Verification items for the finished model (mm, model axes). Face numbers are marked on the shaded views. Round coordinates to 2 decimals unless told otherwise and drop trailing zeros. Order: outer loops, then holes, each group sorted by start corner. A loop starts at its lowest first (then second) coordinate and runs counter-clockwise, first axis right, second up. Notation, with made-up numbers: (41, 74) -> (80, 74) arc R15 cw to (80, 86) -> close; hole circle Ø9 at (-11.75, 23). An arc over 180 degrees is marked (long way). Return JSON: item names as keys, results as strings. Group by question number.
Item 1: Sectioned sample at B-B on x = 32. Record the cut outline in (y, z).
Item 2: Scan lines: probe 1 along Y at (x, z) = (32, -1.25); probe 2 along X at (y, z) = (17, -1.5); probe 3 along Z at (x, y) = (67.5, 23.5). Record each from-to range of solid material in increasing order. Write a range as from..to.
Item 3: Depth check by flat-ended pin: pin 1 Ø8.5 at (x, y) = (47.5, 13) entering from +Z; pin 2 Ø4 at (y, z) = (9.5, 1.5) entering from -X. Enter the tip coordinate at first touch or a pass-through.
Item 4: Draft check along X on the marked faces 1 and 2. Enter one of: pulls with the +X half, pulls with the -X half, needs draft (parallel to the pull), parting line crosses it, or undercut.
Item 5: Sectioned sample at A-A on y = 15. Record the cut outline in (x, z).
Item 6: Sectioned sample at C-C on y = 24.75. Record the cut outline in (x, z), plus the area to 3 significant figures.
Item 7: Sectioned sample at D-D on z = 1.25. Record the cut outline in (x, y).
```python
from build123d import *

# Parameters (mm, degrees)
F0_W     = 98
F0_H     = 30
F0_R     = 7.5
F0_R_2   = 2.25
F1_DEPTH = 3
F2_DEPTH = 4
F3_R     = 1.9
F4_R     = 1


with BuildPart() as f1:
    # F0 (on Top) → F1 (new body)
    with BuildSketch(Plane.XY):
        with Locations((49, 15)):
            Rectangle(F0_W, F0_H)
        with Locations((15, 15)):
            Circle(F0_R, mode=Mode.SUBTRACT)
        with Locations((32, 15)):
            Circle(F0_R_2, mode=Mode.SUBTRACT)
        with Locations((66, 15)):
            Circle(F0_R_2, mode=Mode.SUBTRACT)
        with Locations((83, 15)):
            Circle(F0_R, mode=Mode.SUBTRACT)
        with Locations((83, 15)):
            Circle(F0_R)
        with Locations((15, 15)):
            Circle(F0_R)
    extrude(amount=-F1_DEPTH)

    # F0 (on Top) → F2 (join)
    with BuildSketch(Plane.XY):
        with Locations((15, 15)):
            Circle(F0_R)
        with Locations((83, 15)):
            Circle(F0_R)
    extrude(amount=F2_DEPTH)

    # F3
    f3_edges = [f1.edges().sort_by_distance(p)[0] for p in [
        (7.5, 15, 4),
        (75.5, 15, 4),
    ]]
    fillet(f3_edges, radius=F3_R)

    # F4
    f4_edges = [f1.edges().sort_by_distance(p)[0] for p in [
        (49, 30, 0),
        (0, 15, 0),
        (98, 15, 0),
        (49, 0, 0),
    ]]
    fillet(f4_edges, radius=F4_R)


solid = f1.part
```
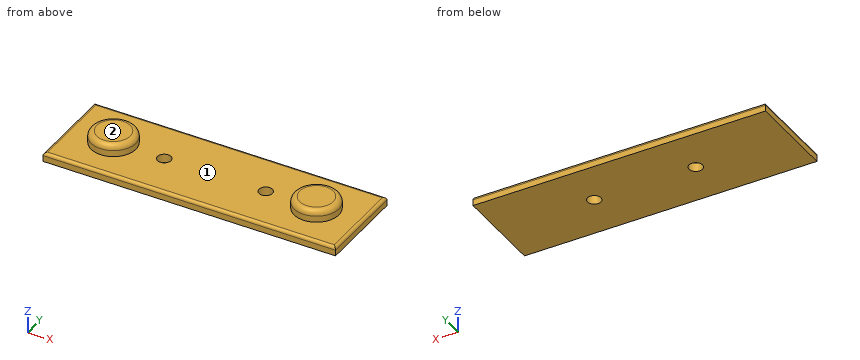
Recorded:
{
 "1": {"outline": "(0, -3) -> (12.75, -3) -> (12.75, 0) -> (1, 0) arc R1 ccw to (0, -1) -> close; (17.25, -3) -> (30, -3) -> (30, -1) arc R1 ccw to (29, 0) -> (17.25, 0) -> close"},
 "2": {"probe 1": "0..12.75, 17.25..30", "probe 2": "0..30.97, 33.03..64.97, 67.03..98", "probe 3": "-3..0"},
 "3": {"pin 1": "z = 0", "pin 2": "x = 0.13"},
 "4": {"face 1": "undercut", "face 2": "needs draft"},
 "5": {"outline": "(0, -3) -> (29.75, -3) -> (29.75, 0) -> (22.5, 0) -> (22.5, 2.1) arc R1.9 ccw to (20.6, 4) -> (9.4, 4) arc R1.9 ccw to (7.5, 2.1) -> (7.5, 0) -> (1, 0) arc R1 ccw to (0, -1) -> close; (34.25, -3) -> (63.75, -3) -> (63.75, 0) -> (34.25, 0) -> close; (68.25, -3) -> (98, -3) -> (98, -1) arc R1 ccw to (97, 0) -> (90.5, 0) -> (90.5, 2.1) arc R1.9 ccw to (88.6, 4) -> (77.4, 4) arc R1.9 ccw to (75.5, 2.1) -> (75.5, 0) -> (68.25, 0) -> close"},
 "6": {"outline": "(0, -3) -> (98, -3) -> (98, -1) arc R1 ccw to (97, 0) -> (1, 0) arc R1 ccw to (0, -1) -> close", "area": "294 mm²"},
 "7": {"outline": "circle Ø15 at (15, 15); circle Ø15 at (83, 15)"}
}
